Could you check a few things on this model? Use its own coordinates, in mm. A direction names the side the tool comes from. Round coordinates to 2 decimals unless told otherwise and drop trailing zeros. Write each loop counter-clockwise with the first axis right and the second up, starting at its lowest first coordinate (ties: lowest second). Pieces come first, ordered by that corner, then holes. Notation, with made-up numbers: (76.25, 57.25) - (93.25, 57.25) arc R21 ccw to (93.25, 92.25) - close; hole circle Ø9 at (-39, 23.5). An arc over 180 degrees is marked (long way). Write each question's results on one line, items separated by ' | '. Start each with the question number.
(1) Imagine slicing it at A-A on z = -3. Write out the boundary of the cut face in (x, y), then the cut area to 3 significant figures.
(2) Imagine slicing it at B-B on x = -6. Write out the boundary of the cut face in (y, z).
(3) Imagine slicing it at C-C on y = 37.5. Write out the boundary of the cut face in (x, z), then the cut area to 3 significant figures.
(4) Imagine slicing it at D-D on x = -1. Write out the boundary of the cut face in (y, z), then the cut area to 3 significant figures.
(5) Thinking about a two-plate mould opening in Z: for faces 1 (the cylindrical face through (8.65, 20.12, 16.12)), 2 (the flat face through (-0.1, 35.65, 7.16)), 3 (the flat face through (-16.85, 17, 5)), which applies, +Z half, -Z half, draft (parallel to the pull), parting line (faces both ways), or undercut?
(6) Please list where these lines run through material, in increasing order: line 1 (X direction, y = 21, z = -4); line 2 (Y direction, x = 10, z = 8); line 3 (X direction, y = 6, z = 14.5). Write a range as [from, to].
(7) For P1, Ø4, axis at y = 12.5, z = -6.5, coming from the -X side; P2, Ø2, axis at x = -13.5, z = 5.5, coming from the +Y side; P3, Ø4, axis at x = 6, z = -3, coming from the +Y side; P4, Ø1, axis at x = 1, z = -9.5, coming from the -Y side, each with a flat end and sliding along its axis, tell me the tip position at first contact or that it passes through.
(8) On a 3-axis mill with a long thin cutter (end or side, diameter ignored), from which of +Z, -Z, +X, -X, +Y, -Y can I reach the whole of each face in a straight line? I mean faces 4 (the flat face through (0, 16.85, -9)), 5 (the flat face through (-0.729, 18.197, 15.475)), 6 (the flat face through (-8.26, 34.77, 7.66)), 7 (the flat face through (-9.15, 0, 10)), 8 (the flat face through (-12, 4, 0)). Say none if no direction works.
```python
from build123d import *

# Parameters (mm, degrees)
PAD_DEPTH       = 20
POCKET_DEPTH    = 35
POCKET001_DEPTH = 25
POCKET002_DEPTH = 30
SKETCH004_W     = 23
SKETCH004_H     = 30
POCKET003_DEPTH = 5
PAD001_DEPTH    = 10
POCKET004_DEPTH = 35
SKETCH007_R     = 3.25
SKETCH007_R_2   = 1.75
POCKET005_DEPTH = 5
CHAMFER_SIZE    = 0.9
PAD002_DEPTH    = 2


with BuildPart() as part:
    # Sketch → Pad (new body)
    with BuildSketch(Plane.XY):
        with BuildLine():
            ThreePointArc((-16.85, 0), (-12, -4.85), (-7.15, 0))
            Line((-7.15, 0), (-7.15, 10))
            ThreePointArc((7.15, 10), (0, 15.4244528418), (-7.15, 10))
            Line((7.15, 0), (7.15, 10))
            ThreePointArc((7.15, 0), (12, -4.85), (16.85, 0))
            Line((16.85, 0), (16.85, 35))
            ThreePointArc((16.85, 35), (15.4294678888, 38.4294678888), (12, 39.85))
            Line((-12, 39.85), (12, 39.85))
            ThreePointArc((-12, 39.85), (-15.4294678888, 38.4294678888), (-16.85, 35))
            Line((-16.85, 0), (-16.85, 35))
        make_face()
        Polygon((-9.15, -1.6454482672), (-9.15, 1.6454482672), (-12, 3.2908965344), (-14.85, 1.6454482672), (-14.85, -1.6454482672), (-12, -3.2908965344), align=None, mode=Mode.SUBTRACT)
        Polygon((14.85, -1.6454482672), (14.85, 1.6454482672), (12, 3.2908965344), (9.15, 1.6454482672), (9.15, -1.6454482672), (12, -3.2908965344), align=None, mode=Mode.SUBTRACT)
    extrude(amount=PAD_DEPTH)

    # Sketch001 (on Face8 of Pad) → Pocket (cut)
    with BuildSketch(Plane.YZ.offset(16.85)):
        Polygon((7.6987298108, 25), (51, 25), (51, 0), align=None)
    extrude(amount=-POCKET_DEPTH, mode=Mode.SUBTRACT)

    # Sketch002 (on Face4 of Pocket) → Pocket001 (cut)
    with BuildSketch(Plane(origin=(0, 12.75, 22.0836477965), x_dir=(1, 0, 0), z_dir=(0, 0.5, 0.8660254038))):
        with BuildLine():
            Line((-7.25, 27.2923845901), (7.25, 27.2923845901))
            ThreePointArc((9.25, 25.2923845901), (8.6642135624, 26.7065981525), (7.25, 27.2923845901))
            Line((9.25, 25.2923845901), (9.25, 10.7923845901))
            ThreePointArc((7.25, 8.7923845901), (8.6642135624, 9.3781710277), (9.25, 10.7923845901))
            Line((-7.25, 8.7923845901), (7.25, 8.7923845901))
            ThreePointArc((-9.25, 10.7923845901), (-8.6642135624, 9.3781710277), (-7.25, 8.7923845901))
            Line((-9.25, 25.2923845901), (-9.25, 10.7923845901))
            Line((-9.25, 25.2923845901), (-7.25, 27.2923845901))
        make_face()
    extrude(amount=-POCKET001_DEPTH, mode=Mode.SUBTRACT)

    # Sketch003 (on DatumPlane) → Pocket002 (cut)
    with BuildSketch(Plane(origin=(0, 12.1160254038, 18.9855715851), x_dir=(1, 0, 0), z_dir=(0, 0.5, 0.8660254038))):
        Polygon((-10.5, 28.2923845901), (10.5, 28.2923845901), (10.5, 5.2923845901), (5, 5.2923845901), (5, -0.7076154099), (-5, -0.7076154099), (-5, 5.2923845901), (-10.5, 5.2923845901), align=None)
    extrude(amount=-POCKET002_DEPTH, mode=Mode.SUBTRACT)

    # Sketch004 (on Face2 of Pocket002) → Pocket003 (cut)
    with BuildSketch(Plane(origin=(0, 0, 0), x_dir=(1, 0, 0), z_dir=(0, 0, -1))):
        with Locations((0, -21.85)):
            Rectangle(SKETCH004_W, SKETCH004_H)
    extrude(amount=-POCKET003_DEPTH, mode=Mode.SUBTRACT)

    # Sketch005 (on Face2 of Pocket003) → Pad001 (join)
    with BuildSketch(Plane(origin=(0, 0, 0), x_dir=(1, 0, 0), z_dir=(0, 0, -1))):
        with BuildLine():
            Line((-11.5, -6.85), (-16.85, -6.85))
            Line((-16.85, -6.85), (-16.85, -35))
            ThreePointArc((-16.85, -35), (-15.4294678888, -38.4294678888), (-12, -39.85))
            Line((-12, -39.85), (12, -39.85))
            ThreePointArc((12, -39.85), (15.4294678888, -38.4294678888), (16.85, -35))
            Line((16.85, -6.85), (16.85, -35))
            Line((11.5, -6.85), (16.85, -6.85))
            Line((11.5, -36.85), (11.5, -6.85))
            Line((-11.5, -36.85), (11.5, -36.85))
            Line((-11.5, -6.85), (-11.5, -36.85))
        make_face()
    extrude(amount=PAD001_DEPTH)

    # Sketch006 (on Face25 of Pad001) → Pocket004 (cut)
    with BuildSketch(Plane.YZ.offset(16.85)):
        Polygon((6.85, 0), (16.85, -10), (6.85, -10), align=None)
    extrude(amount=-POCKET004_DEPTH, mode=Mode.SUBTRACT)

    # Sketch007 (on Face7 of Pocket004) → Pocket005 (cut)
    with BuildSketch(Plane(origin=(0, 39.85, 0), x_dir=(-1, 0, 0), z_dir=(0, 1, 0))):
        with Locations((0, -3)):
            Circle(SKETCH007_R)
        with Locations((6, -3)):
            Circle(SKETCH007_R_2)
        with Locations((-6, -3)):
            Circle(SKETCH007_R_2)
    extrude(amount=-POCKET005_DEPTH, mode=Mode.SUBTRACT)

    # Chamfer
    chamfer_edges = [part.edges().sort_by_distance(p)[0] for p in [
        (7.75, 39.85, -3),
        (-4.25, 39.85, -3),
    ]]
    chamfer(chamfer_edges, length=CHAMFER_SIZE)

    # Sketch008 (on Face8 of Pocket005) → Pad002 (join)
    with BuildSketch(Plane(origin=(0, 0, -10), x_dir=(1, 0, 0), z_dir=(0, 0, -1))):
        with BuildLine():
            Line((-16.85, -16.85), (16.85, -16.85))
            Line((16.85, -16.85), (16.85, -35))
            ThreePointArc((12, -39.85), (15.4294678888, -38.4294678888), (16.85, -35))
            Line((12, -39.85), (-12, -39.85))
            ThreePointArc((-16.85, -35), (-15.4294678888, -38.4294678888), (-12, -39.85))
            Line((-16.85, -16.85), (-16.85, -35))
        make_face()
    extrude(amount=-PAD002_DEPTH)


solid = part.part
```
Response:
1) outline: (-16.85, 9.85) - (-11.5, 9.85) - (-11.5, 36.85) - (-7.75, 36.85) - (-7.75, 38.95) - (-8.65, 39.85) - (-12, 39.85) arc R4.85 ccw to (-16.85, 35) - close; (-4.25, 36.85) - (-3.25, 36.85) - (-3.25, 39.85) - (-3.35, 39.85) - (-4.25, 38.95) - close; (3.25, 36.85) - (4.25, 36.85) - (4.25, 38.95) - (3.35, 39.85) - (3.25, 39.85) - close; (7.75, 36.85) - (11.5, 36.85) - (11.5, 9.85) - (16.85, 9.85) - (16.85, 35) arc R4.85 ccw to (12, 39.85) - (8.65, 39.85) - (7.75, 38.95) - close | area: 338 mm²
2) outline: (12.37, 8.85) - (16.7, 16.34) - (18.86, 15.09) - (20.36, 17.69) - (16.36, 20) - (12.37, 20) - close; (16.85, -10) - (39.85, -10) - (39.85, -5.65) - (38.95, -4.75) - (36.85, -4.75) - (36.85, -8) - (16.85, -8) - close; (34.89, 5.84) - (36.34, 5) - (36.85, 5) - (36.85, -1.25) - (38.95, -1.25) - (39.85, -0.35) - (39.85, 6.44) - (36.39, 8.44) - close
3) outline: (-16.16, -10) - (16.16, -10) - (16.16, 7.79) - (-16.16, 7.79) - close; hole circle Ø3.5 at (-6, -3); hole circle Ø6.5 at (0, -3); hole circle Ø3.5 at (6, -3) | area: 523 mm²
4) outline: (15.36, 17.11) - (18.86, 15.09) - (20.36, 17.69) - (16.36, 20) - (15.36, 20) - close; (16.85, -10) - (39.85, -10) - (39.85, -6.09) - (36.85, -6.09) - (36.85, -8) - (16.85, -8) - close; (34.89, 5.84) - (36.34, 5) - (36.85, 5) - (36.85, 0.09) - (39.85, 0.09) - (39.85, 6.44) - (36.39, 8.44) - close | area: 91.9 mm²
5) face 1: undercut | face 2: +Z half | face 3: draft
6) line 1: [-16.85, -11.5], [11.5, 16.85] | line 2: [-4.42, -2.14], [2.14, 11.88], [31.14, 37.14] | line 3: [-16.85, -7.15], [7.15, 16.85]
7) P1: x = -16.85 | P2: y = 39.82 | P3: y = 39.2 | P4: y = 16.85
8) face 4: -Z, -Y | face 5: none | face 6: +Z | face 7: +Z, -Z | face 8: -Z, +X, -X, -Y
